The listing builds one solid part. Answer for the finished solid, in the listing's coordinates (mm). Round coordinates to 2 decimals unless told otherwise and drop trailing zeros. Write each loop counter-clockwise with the first axis right and the second up, starting at its lowest first coordinate (ties: lowest second). Pieces come first, ordered by that corner, then holes. Notation, with made-up numbers: (63.25, -28.5) - (116.25, -28.5) arc R22 cw to (116.25, -15.5) - close; hole circle Ø5 at (-5.5, 32). An arc over 180 degrees is marked (long way). Answer as CSV lines item,"result". Start each with the question number.
Item 1: A cutting plane is placed at A-A on y = 2.4. State how many separate pieces and enclosed holes the cut face has, and give its area (3 significant figures).
Item 2: A cutting plane is placed at B-B on x = -245. Determine the outline of the cut face in (y, z) (3 decimals).
Item 3: Straight lines are drawn through the part: line 1 along Z through (x, y) = (878, 1.5); line 2 along Z through (x, y) = (36, 2.2); line 3 along Z through (x, y) = (402, 0.7). For each, find the intervals that lie inside material, in ascending order. Write a range as [from, to].
Item 4: A cutting plane is placed at C-C on z = -416.5. Determine the outline of the cut face in (x, y) (3 decimals).
Item 5: Flat-ended cylindrical pins translate along their axes: pin 1 (7.5 mm diameter, centred on x = 511.34, z = -464.87, fed in from -Y); pin 2 (1 mm diameter, centred on y = 2, z = -118.5, fed in from +X); pin 3 (14.5 mm diameter, centred on x = 434.69, z = -496.62, fed in from -Y); pin 4 (1.6 mm diameter, centred on x = 826, y = 1.5, fed in from +Z). Find the tip coordinate at first contact, or state that the pin passes through.
```python
from build123d import *

# Parameters (mm, degrees)
SKETCH2_R           = 6.35
SKETCH2_R_2         = 2.45745
BOSS_EXTRUDE1_DEPTH = 3.175


with BuildPart() as part:
    # Sketch2 → Boss-Extrude1 (new body)
    with BuildSketch(Plane(origin=(0, 0, 0), x_dir=(1, 0, 0), z_dir=(0, 1, 0))):
        with BuildLine():
            ThreePointArc((-523.9004, 138.064786013), (-521.881202428, 132.200610461), (-516.679706056, 128.82271922))
            Line((-516.679706056, 128.82271922), (-1.134783113, 0.282933207))
            ThreePointArc((-1.134783113, 0.282933207), (0.008717447, 0.070997906), (1.169522943, 0))
            Line((1.169522943, 0), (122.844814136, 0))
            Line((122.844814136, 0), (122.844814136, 88.9))
            Line((122.844814136, 88.9), (175.168814136, 88.9))
            Line((175.168814136, 88.9), (175.168814136, 0))
            Line((175.168814136, 0), (351.444814136, 0))
            Line((351.444814136, 0), (351.444814136, 88.9))
            Line((351.444814136, 88.9), (403.768814136, 88.9))
            Line((403.768814136, 88.9), (403.768814136, 0))
            Line((403.768814136, 0), (580.044814136, 0))
            Line((580.044814136, 0), (580.044814136, 88.9))
            Line((580.044814136, 88.9), (632.368814136, 88.9))
            Line((632.368814136, 88.9), (632.368814136, 0))
            Line((632.368814136, 0), (808.644814136, 0))
            Line((808.644814136, 0), (808.644814136, 88.9))
            Line((808.644814136, 88.9), (860.968814136, 88.9))
            Line((860.968814136, 88.9), (860.968814136, 0))
            Line((860.968814136, 0), (973.929215818, 0))
            ThreePointArc((973.929215818, 0), (982.729168366, 5.879940307), (980.664407909, 16.260192091))
            Line((980.664407909, 16.260192091), (491.714407909, 505.210192091))
            ThreePointArc((491.714407909, 505.210192091), (488.624275512, 507.274952547), (484.979215818, 508))
            Line((484.979215818, 508), (-78.566585303, 508))
            ThreePointArc((-78.566585303, 508), (-80.220584195, 507.855293847), (-81.824327168, 507.425572213))
            Line((-81.824327168, 507.425572213), (-517.633141865, 348.804135832))
            ThreePointArc((-517.633141865, 348.804135832), (-522.177823222, 345.316879176), (-523.9004, 339.853563619))
            Line((-523.9004, 339.853563619), (-523.9004, 138.064786013))
        make_face()
        with Locations((1.976178059, 15.875)):
            Circle(SKETCH2_R, mode=Mode.SUBTRACT)
        with Locations((-125.36611658, 47.625)):
            Circle(SKETCH2_R, mode=Mode.SUBTRACT)
        with Locations((5.874587868, 47.625)):
            Circle(SKETCH2_R, mode=Mode.SUBTRACT)
        with Locations((-476.2754, 135.116510814)):
            Circle(SKETCH2_R, mode=Mode.SUBTRACT)
        with Locations((-508.0254, 143.032674904)):
            Circle(SKETCH2_R, mode=Mode.SUBTRACT)
        with Locations((-476.2754, 167.838493546)):
            Circle(SKETCH2_R, mode=Mode.SUBTRACT)
        with Locations((-508.0254, 175.754657636)):
            Circle(SKETCH2_R, mode=Mode.SUBTRACT)
        with Locations((-493.0394, 199.090929312)):
            Circle(SKETCH2_R_2, mode=Mode.SUBTRACT)
        with Locations((263.306814136, 32.385)):
            Circle(SKETCH2_R_2, mode=Mode.SUBTRACT)
        with Locations((491.906814136, 32.385)):
            Circle(SKETCH2_R_2, mode=Mode.SUBTRACT)
        with Locations((720.506814136, 32.385)):
            Circle(SKETCH2_R_2, mode=Mode.SUBTRACT)
        with Locations((877.339781319, 53.975)):
            Circle(SKETCH2_R, mode=Mode.SUBTRACT)
        with Locations((899.564781319, 31.75)):
            Circle(SKETCH2_R, mode=Mode.SUBTRACT)
        with Locations((944.466061924, 31.75)):
            Circle(SKETCH2_R, mode=Mode.SUBTRACT)
        with Locations((922.241061924, 53.975)):
            Circle(SKETCH2_R, mode=Mode.SUBTRACT)
        with Locations((-493.0394, 276.290731215)):
            Circle(SKETCH2_R_2, mode=Mode.SUBTRACT)
        with Locations((-508.0254, 299.333610137)):
            Circle(SKETCH2_R, mode=Mode.SUBTRACT)
        with Locations((-476.2754, 310.889665075)):
            Circle(SKETCH2_R, mode=Mode.SUBTRACT)
        with Locations((-508.0254, 333.121254413)):
            Circle(SKETCH2_R, mode=Mode.SUBTRACT)
        with Locations((-476.2754, 344.677309351)):
            Circle(SKETCH2_R, mode=Mode.SUBTRACT)
        with Locations((-146.038641871, 464.873096997)):
            Circle(SKETCH2_R, mode=Mode.SUBTRACT)
        with Locations((-53.207852166, 464.873081124)):
            Circle(SKETCH2_R, mode=Mode.SUBTRACT)
        with Locations((-58.806228375, 496.623082082)):
            Circle(SKETCH2_R, mode=Mode.SUBTRACT)
        with Locations((34.024561331, 496.623066209)):
            Circle(SKETCH2_R, mode=Mode.SUBTRACT)
        with Locations((102.750499745, 481.637016811)):
            Circle(SKETCH2_R_2, mode=Mode.SUBTRACT)
        with Locations((322.928740552, 481.637016811)):
            Circle(SKETCH2_R_2, mode=Mode.SUBTRACT)
        with Locations((466.441944838, 464.872992272)):
            Circle(SKETCH2_R, mode=Mode.SUBTRACT)
        with Locations((511.343225443, 464.872984595)):
            Circle(SKETCH2_R, mode=Mode.SUBTRACT)
        with Locations((434.691950267, 496.622997701)):
            Circle(SKETCH2_R, mode=Mode.SUBTRACT)
        with Locations((479.593230872, 496.622990024)):
            Circle(SKETCH2_R, mode=Mode.SUBTRACT)
    extrude(amount=BOSS_EXTRUDE1_DEPTH)


solid = part.part
```
Geometry says:
1,separate pieces,"1"
1,enclosed holes,"30"
1,area,"552,000 mm^2"
2,outline,"(0, -448.034) - (3.175, -448.034) - (3.175, -61.085) - (0, -61.085) - close"
3,line 1,"z = [-118.92, -60.29], [-47.66, 0]"
3,line 2,"z = [-508, -502.66], [-490.59, 0]"
3,line 3,"z = [-508, -88.9]"
4,outline,"(-331.64, 0) - (580.425, 0) - (580.425, 3.175) - (-331.64, 3.175) - close"
5,pin 1,"passes through"
5,pin 2,"stops at x = 878.92"
5,pin 3,"stops at y = 0"
5,pin 4,"stops at z = -88.9"
